For this review, take the finished solid that the model builds, in its own axes (mm). A direction names the side the tool comes from. Give positions to 0.01 mm unless a question says otherwise; leave off trailing zeros. Order: outer loops, then holes, each group sorted by start corner. A loop starts at its lowest first (then second) coordinate and runs counter-clockwise, first axis right, second up. Notation, with made-up numbers: (10.25, 71) -> (29.25, 71) arc R23 cw to (29.25, 83) -> close; hole circle Ø2 at (88, -19). An arc over 180 degrees is marked (long way). One line per item, written item: value. Start each with the question number.
from build123d import *

# Parameters (mm, degrees)
CYLINDER001_R     = 4
CYLINDER001_DEPTH = 10
CYLINDER_R        = 5
CYLINDER_DEPTH    = 10


with BuildPart() as con001:
    # Cone001 → Cone001 (revolve)
    with BuildSketch(Plane.XZ):
        Polygon((0, 0), (4, 0), (24, 30), (0, 30), align=None)
    revolve(axis=Axis((0, 0, 0), (0, 0, 1)))


with BuildPart() as cut:
    # Cone → Cone (revolve)
    with BuildSketch(Plane.XZ):
        Polygon((0, 0), (5, 0), (25, 30), (0, 30), align=None)
    revolve(axis=Axis((0, 0, 0), (0, 0, 1)))

    # Cut: cut Con001
    add(con001.part, mode=Mode.SUBTRACT)


with BuildPart() as cilindre001:
    # Cylinder001 → Cylinder001 (new body)
    with BuildSketch(Plane.XY.offset(-10)):
        Circle(CYLINDER001_R)
    extrude(amount=CYLINDER001_DEPTH)


with BuildPart() as obj1:
    # Cylinder → Cylinder (new body)
    with BuildSketch(Plane.XY.offset(-10)):
        Circle(CYLINDER_R)
    extrude(amount=CYLINDER_DEPTH)

    # Cut001: cut Cilindre001
    add(cilindre001.part, mode=Mode.SUBTRACT)

    # Fusion: union Cut
    add(cut.part)


solid = obj1.part
Q1. For line 1 along Y through (x, z) = (0, -2); line 2 along Y through (x, z) = (10.5, 21.5); line 3 along X through (y, z) = (7, 12), list the stretches that pass through material, from the lowest coordinate up.
Q2. Mouldability with a two-part tool opening along Y and no side actions: class faces 1 (the flat face through (-9.4, 22.3, 30)), 2 (the cylindrical face through (-0.867, -3.905, -5.07)), 3 (the conical face through (10.2, 3.21, 8.54)) as pulls with the +Y half, pulls with the -Y half, needs draft (parallel to the pull), parting line crosses it, or undercut.
Q3. For pin 1 Ø6 at (x, y) = (-4, 18.5) entering from +Z; pin 2 Ø4 at (y, z) = (-11.5, 21) entering from +X; pin 3 Ø2 at (x, y) = (4.5, -15.5) entering from -Z, all flat-tipped, find the tip position at first contact; note any pin that passes through.
Q4. For faces 4 (the cylindrical face through (-1.08, -4.88, -5.07)), 5 (the conical face through (9.248, 2.912, 8.543)), list the 3-axis set-ups (+Z, -Z, +X, -X, +Y, -Y) from which the entire face can be reached by the end or side of a thin tool; tool diameter is ignored.
Q5. Take a section at D-D (z = 13). State the section outline as (x, y) points.
Q6. Take a section at C-C (z = -5). State the section outline as (x, y) points.
Q7. Take a section at A-A (y = 0). State the section outline as (x, z) points, and give its area (3 significant figures).
Answers below:
1. line 1: y = -5 to -4, 4 to 5
1. line 2: y = -16.23 to -15.03, 15.03 to 16.23
1. line 3: x = -10.95 to -9.75, 9.75 to 10.95
2. face 1: needs draft
2. face 2: undercut
2. face 3: parting line crosses it
3. pin 1: stops at z = 26.89
3. pin 2: stops at x = 17.22
3. pin 3: stops at z = 15.21
4. face 4: -Z
4. face 5: +Z
5. outline: circle Ø27.33 at (0, 0); hole circle Ø25.33 at (0, 0)
6. outline: circle Ø10 at (0, 0); hole circle Ø8 at (0, 0)
7. outline: (-25, 30) -> (-5, 0) -> (-5, -10) -> (-4, -10) -> (-4, 0) -> (-24, 30) -> close; (4, -10) -> (5, -10) -> (5, 0) -> (25, 30) -> (24, 30) -> (4, 0) -> close
7. area: 80.0 mm²
